Check sheet for the modelled part. Datum: model origin and axes. Units: mm. A direction names the side the tool comes from. Round coordinates to 2 decimals unless told otherwise and drop trailing zeros. One line per question, with ' | ' between items. Start each with the question number.
(1) Tool access check on faces 1 (the face through (-224, 8, -14)), 2 (the face through (198, 8, -39)), 3 (the face through (-250, 8, -259)). Record the directions out of +Z, -Z, +X, -X, +Y, -Y that give a thin tool (end or side, any length) a straight path to the whole face; none if there is none.
(2) Draft check along Z on faces 4 (the face through (-212.5, 8, -189)), 5 (the face through (-3, 8, 310)), 6 (the face through (250, 8, -115)). Enter one of: +Z half, -Z half, draft (parallel to the pull), parting line (faces both ways), or undercut.
(3) Thickness scan on probe 1 along X at (y, z) = (4.5, 124.5). Record the ranges inside material, lowest first. Write a range as [from, to].
(4) Go/stop test with flat-tipped pins: P1, Ø3, axis at y = 13, z = -59, coming from the +X side; P2, Ø5, axis at y = 8, z = 107.5, coming from the -X side; P3, Ø5.5, axis at y = 10, z = 95, coming from the +X side; P4, Ø8, axis at x = 46, z = -59, coming from the -Y side. Record where each tip stops, or that it passes through.
```python
from build123d import *

# Parameters (mm, degrees)
SKETCH1_W           = 500
SKETCH1_H           = 620
BOSS_EXTRUDE1_DEPTH = 16.5
SKETCH2_W           = 52
SKETCH2_H           = 50
CUT_EXTRUDE1_DEPTH  = 17.5


with BuildPart() as part:
    # Sketch1 → Boss-Extrude1 (new body)
    with BuildSketch(Plane(origin=(0, 0, 0), x_dir=(1, 0, 0), z_dir=(0, 1, 0))):
        Rectangle(SKETCH1_W, SKETCH1_H)
    extrude(amount=BOSS_EXTRUDE1_DEPTH)

    # Sketch2 → Cut-Extrude1 (cut, through all)
    with BuildSketch(Plane(origin=(0, 16.5, 0), x_dir=(1, 0, 0), z_dir=(0, 1, 0))):
        with Locations((-224, 39)):
            Rectangle(SKETCH2_W, SKETCH2_H)
        with Locations((224, 39)):
            Rectangle(SKETCH2_W, SKETCH2_H)
        Polygon((-250, 210), (-244, 210), (-244, 199), (-212.5, 199), (-212.5, 179), (-244, 179), (-244, 168), (-250, 168), align=None)
        Polygon((212.5, 199), (212.5, 179), (244, 179), (244, 168), (250, 168), (250, 210), (244, 210), (244, 199), align=None)
        Polygon((212.5, -101), (212.5, -121), (244, -121), (244, -132), (250, -132), (250, -90), (244, -90), (244, -101), align=None)
        Polygon((-250, -90), (-244, -90), (-244, -101), (-212.5, -101), (-212.5, -121), (-244, -121), (-244, -132), (-250, -132), align=None)
    extrude(amount=-CUT_EXTRUDE1_DEPTH, mode=Mode.SUBTRACT)


solid = part.part
```
The answers:
1) face 1: -X, +Y, -Y | face 2: +X, +Y, -Y | face 3: +Z, -Z, -X, +Y, -Y
2) face 4: undercut | face 5: +Z half | face 6: draft
3) probe 1: [-244, 244]
4) P1: x = 198 | P2: x = -212.5 | P3: x = 244 | P4: y = 0
